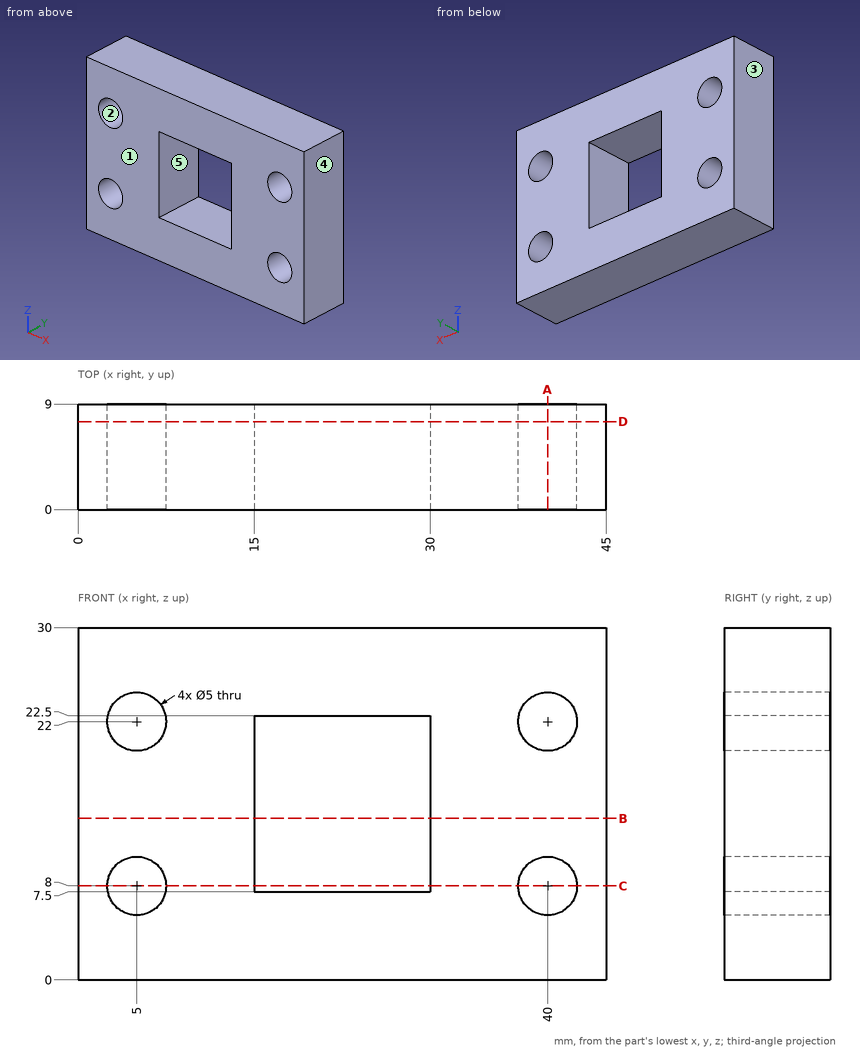
Source: three-view drawing plus pictorial views. Frame: mm from the lowest corner of the part. A direction names the side the tool comes from. Coordinates: 2 decimals unless noted, no trailing zeros. Loops run counter-clockwise (first coordinate to the right, second up) from the corner with the lowest first, then second, coordinate; pieces in that order, holes last. Notation, with made-up numbers: (-36, -26.75) - (7, -26.75) arc R17 cw to (7, 4.25) - close; hole circle Ø6 at (-28, 67.25). An arc over 180 degrees is marked (long way). One line per question, with ' | ' between items.
1) Section D-D, the plane y = 7.5. Return loops of the section in (x, z).
Report:
outline: (0, 0) - (45, 0) - (45, 30) - (0, 30) - close; hole circle Ø5 at (5, 8); hole circle Ø5 at (5, 22); hole (15, 7.5) - (30, 7.5) - (30, 22.5) - (15, 22.5) - close; hole circle Ø5 at (40, 8); hole circle Ø5 at (40, 22)
2) First-contact query: P1, Ø2, axis at x = 18, z = 25.5, coming from the -Y side. Flat tip, straight axial feed; report the tip coordinate or a pass-through.
Report:
P1: stops at y = 0
3) Section C-C, the plane z = 8. Return loops of the section in (x, y).
Report:
outline: (0, 0) - (2.5, 0) - (2.5, 9) - (0, 9) - close; (7.5, 0) - (15, 0) - (15, 9) - (7.5, 9) - close; (30, 0) - (37.5, 0) - (37.5, 9) - (30, 9) - close; (42.5, 0) - (45, 0) - (45, 9) - (42.5, 9) - close
4) Set-up query: the marked faces 4 and 5. Return all of +Z, -Z, +X, -X, +Y, -Y with unobstructed straight access to the full face (end or side cutting, diameter ignored); none if empty.
Report:
face 4: +Z, -Z, +X, +Y, -Y | face 5: +Y, -Y
5) Section A-A, the plane x = 40. Return loops of the section in (y, z).
Report:
outline: (0, 0) - (9, 0) - (9, 5.5) - (0, 5.5) - close; (0, 10.5) - (9, 10.5) - (9, 19.5) - (0, 19.5) - close; (0, 24.5) - (9, 24.5) - (9, 30) - (0, 30) - close
6) Pull-direction query (X, two-part tool) for the marked faces 1, 2 and 3; classes: released by +X, released by -X, zero draft, split by the parting line, or undercut.
Report:
face 1: zero draft | face 2: undercut | face 3: released by -X
7) Line query: line 1 along X through (y, z) = (3.5, 22); line 2 along Z through (x, y) = (40, 3.5); line 3 along Z through (x, y) = (28, 6.5). Output: solid intervals per line, ascending.
Report:
line 1: x = 0 to 2.5, 7.5 to 15, 30 to 37.5, 42.5 to 45 | line 2: z = 0 to 5.5, 10.5 to 19.5, 24.5 to 30 | line 3: z = 0 to 7.5, 22.5 to 30
8) Section B-B, the plane z = 13.75. Return loops of the section in (x, y).
Report:
outline: (0, 0) - (15, 0) - (15, 9) - (0, 9) - close; (30, 0) - (45, 0) - (45, 9) - (30, 9) - close
